Input: part model. Units: mm. Frame: model coordinates. Face numbers are marked on the shaded views. A direction names the side the tool comes from. Round coordinates to 2 decimals unless told otherwise and drop trailing zeros. Write each loop counter-clockwise with the first axis right and the second up, starting at its lowest first coordinate (ties: lowest second). Pieces come first, ordered by that corner, then holes. Notation, with made-up numbers: (35, 29) -> (60, 29) arc R18 ccw to (60, 57) -> close; hole circle Ø1 at (-13, 47.25). An arc over 180 degrees is marked (long way). Write item = value, one per line. Start each with the question number.
```python
from build123d import *

# Parameters (mm, degrees)
SKETCH1_W               = 68
SKETCH1_H               = 30
BOSS_EXTRUDE1_DEPTH     = 5
SKETCH2_R               = 17.5
BOSS_EXTRUDE2_DEPTH     = 5
SKETCH3_R               = 2.5
CUT_EXTRUDE1_DEPTH      = 1
CUT_EXTRUDE1_DEPTH_BACK = 6


with BuildPart() as part:
    # Sketch1 → Boss-Extrude1 (new body)
    with BuildSketch(Plane(origin=(0, 0, 0), x_dir=(1, 0, 0), z_dir=(0, 1, 0))):
        Rectangle(SKETCH1_W, SKETCH1_H)
    extrude(amount=BOSS_EXTRUDE1_DEPTH)

    # Sketch2 → Boss-Extrude2 (add)
    with BuildSketch(Plane(origin=(0, 5, 0), x_dir=(1, 0, 0), z_dir=(0, 1, 0))):
        with Locations((0, 15)):
            Circle(SKETCH2_R)
    extrude(amount=-BOSS_EXTRUDE2_DEPTH)

    # Sketch3 → Cut-Extrude1 (cut, two sides)
    with BuildSketch(Plane(origin=(0, 5, 0), x_dir=(1, 0, 0), z_dir=(0, 1, 0))) as cut_extrude1_sk:
        with Locations((0, 15)):
            Circle(SKETCH3_R)
    extrude(amount=CUT_EXTRUDE1_DEPTH, mode=Mode.SUBTRACT)
    extrude(cut_extrude1_sk.sketch, amount=-CUT_EXTRUDE1_DEPTH_BACK, mode=Mode.SUBTRACT)


solid = part.part
```
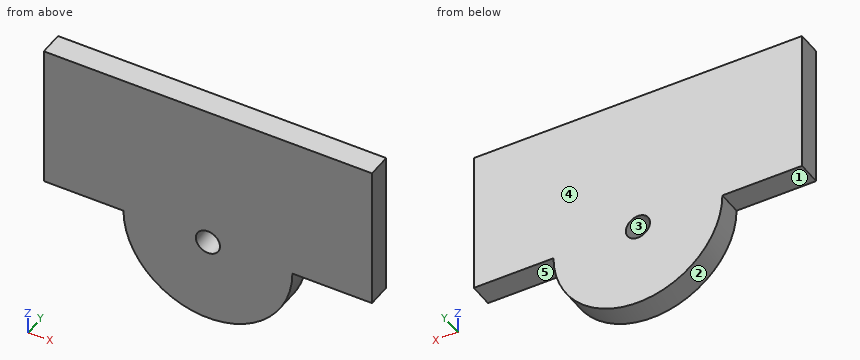
1. Section B-B (y = 4.3). Output: boundary loops of the cut face in (x, z), then the cut area to 3 significant figures.
2. Section C-C (x = -22). Output: boundary loops of the cut face in (y, z), then the cut area to 3 significant figures.
3. Section D-D (z = -21.5). Output: boundary loops of the cut face in (x, y).
4. Mould query, pull axis X, two halves, no side actions, for the marked faces 1, 2 and 3. Classes: pulls with the +X half, pulls with the -X half, needs draft (parallel to the pull), parting line crosses it, or undercut.
5. Section A-A (x = 0). Output: boundary loops of the cut face in (y, z).
6. Pin query (flat end, axial travel): P1, Ø2.5, axis at x = -25, y = 1.5, coming from the -Z side; P2, Ø3, axis at x = -12.5, y = 1, coming from the -Z side. Return the tip coordinate at first contact, or that it passes through.
7. Reachability of the marked faces 4 and 5 from +Z, -Z, +X, -X, +Y, -Y: full face, straight path, thin tool, end or side. Return the list, or none.
8. Line query: line 1 along Z through (x, y) = (0, 1.8); line 2 along Z through (x, y) = (-22, 0.9); line 3 along Z through (x, y) = (-1.5, 0.5). Output: solid intervals per line, ascending.
Check sheet entries:
q1.outline = (-34, -15) -> (-17.5, -15) arc R17.5 ccw to (17.5, -15) -> (34, -15) -> (34, 15) -> (-34, 15) -> close; hole circle Ø5 at (0, -15)
q1.area = 2,500 mm2
q2.outline = (0, -15) -> (5, -15) -> (5, 15) -> (0, 15) -> close
q2.area = 150 mm2
q3.outline = (-16.25, 0) -> (16.25, 0) -> (16.25, 5) -> (-16.25, 5) -> close
q4.face_1 = needs draft
q4.face_2 = parting line crosses it
q4.face_3 = undercut
q5.outline = (0, -32.5) -> (5, -32.5) -> (5, -17.5) -> (0, -17.5) -> close; (0, -12.5) -> (5, -12.5) -> (5, 15) -> (0, 15) -> close
q6.P1 = -15
q6.P2 = -28.61
q7.face_4 = +Z, -Z, +X, -X, +Y
q7.face_5 = -Z, +X, +Y, -Y
q8.line_1 = -32.5 to -17.5, -12.5 to 15
q8.line_2 = -15 to 15
q8.line_3 = -32.44 to -17, -13 to 15
